Answer from the drawing. Dimensions are ordinates in mm from the lowest x, y and z of the part. A direction names the side the tool comes from. Coordinates: 2 decimals unless noted, no trailing zeros. Loops run counter-clockwise (first coordinate to the right, second up) from the corner with the lowest first, then second, coordinate; pieces in that order, holes last.
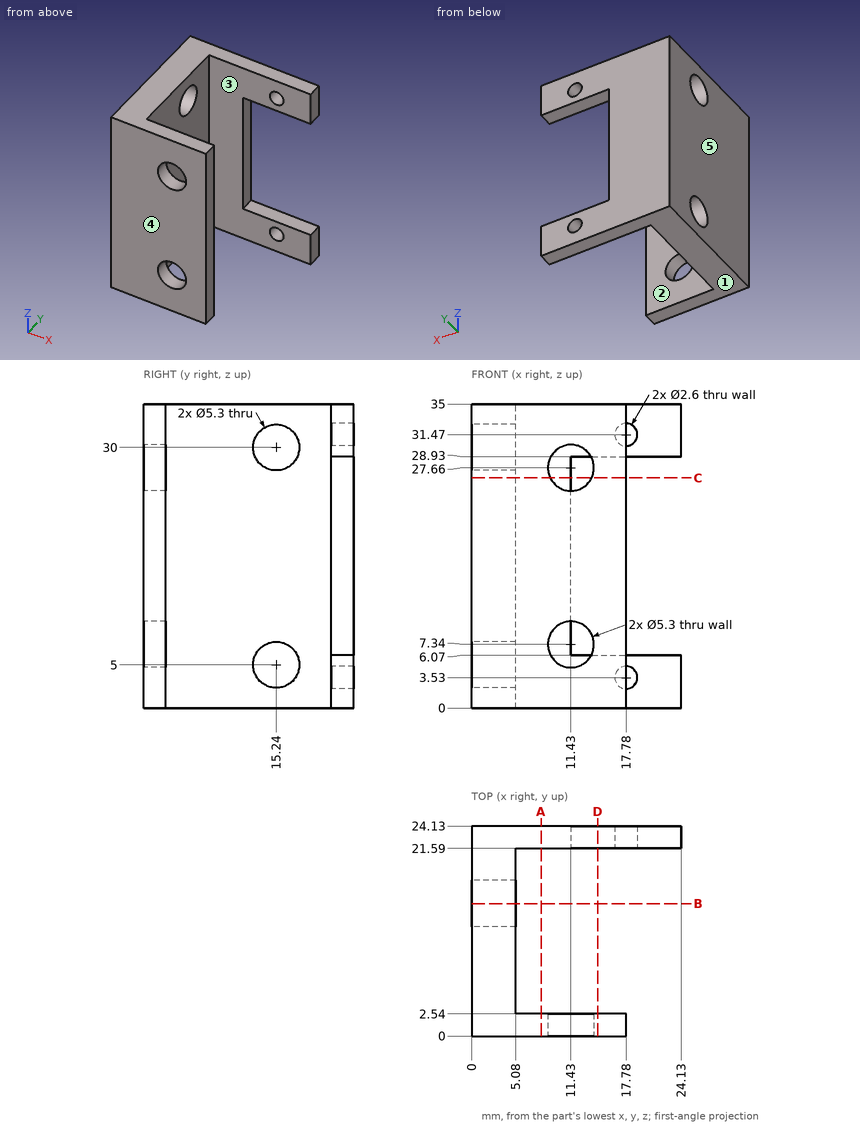
Item 1: A cutting plane is placed at A-A on x = 8. Determine the outline of the cut face in (y, z), then the cut area to 3 significant figures.
Numbers:
outline: (0, 0) - (2.54, 0) - (2.54, 35) - (0, 35) - close; (21.59, 0) - (24.13, 0) - (24.13, 35) - (21.59, 35) - close
area: 178 mm2
Item 2: A cutting plane is placed at D-D on x = 14.5. Determine the outline of the cut face in (y, z), then the cut area to 3 significant figures.
Numbers:
outline: (0, 0) - (2.54, 0) - (2.54, 35) - (0, 35) - close; (21.59, 0) - (24.13, 0) - (24.13, 6.07) - (21.59, 6.07) - close; (21.59, 28.93) - (24.13, 28.93) - (24.13, 35) - (21.59, 35) - close
area: 120 mm2
Item 3: Determine the mould class of the marked faces 3, 4 and 5 for opening direction Y: released by +Y, released by -Y, zero draft, split by the parting line, or undercut.
Numbers:
face 3: undercut
face 4: released by -Y
face 5: zero draft
Item 4: A cutting plane is placed at B-B on y = 15.24. Determine the outline of the cut face in (x, z), then the cut area to 3 significant figures.
Numbers:
outline: (0, 0) - (5.08, 0) - (5.08, 2.35) - (0, 2.35) - close; (0, 7.65) - (5.08, 7.65) - (5.08, 27.35) - (0, 27.35) - close; (0, 32.65) - (5.08, 32.65) - (5.08, 35) - (0, 35) - close
area: 124 mm2
Item 5: Find the intervals of material crossed by line 1 along Z through (x, y) = (17.78, 23); line 2 along Z through (x, y) = (11.43, 0.7); line 3 along X through (y, z) = (9.25, 8), in increasing order.
Numbers:
line 1: z = 0 to 2.23, 4.83 to 6.07, 28.93 to 30.17, 32.77 to 35
line 2: z = 0 to 4.69, 9.99 to 25.01, 30.31 to 35
line 3: x = 0 to 5.08
Item 6: Which of the six approach directions +Z, -Z, +X, -X, +Y, -Y give full straight-line access (tool end or side, diameter ignored) to the marked faces 1 and 2?
Numbers:
face 1: -Z, +X, -X, +Y, -Y
face 2: +Z, -Z, +X
Item 7: A cutting plane is placed at C-C on z = 26.5. Determine the outline of the cut face in (x, y).
Numbers:
outline: (0, 0) - (9.05, 0) - (9.05, 2.54) - (5.08, 2.54) - (5.08, 21.59) - (11.43, 21.59) - (11.43, 24.13) - (0, 24.13) - close; (13.81, 0) - (17.78, 0) - (17.78, 2.54) - (13.81, 2.54) - close
Item 8: Given pin 1 (2 mm diameter, centred on y = 2.5, z = 10, fed in from +X); pin 2 (1.6 mm diameter, centred on x = 17.78, z = 3.53, fed in from +Y); pin 3 (12 mm diameter, centred on y = 12, z = 9, fed in from +X), each flat-ended and moving along its own axis, determine where each tip first touches the part or whether it passes through.
Numbers:
pin 1: stops at x = 17.78
pin 2: stops at y = 2.54
pin 3: stops at x = 5.08
